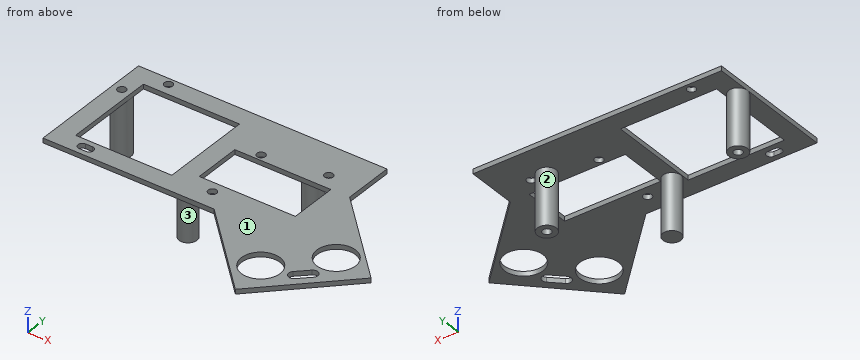
from build123d import *

# Parameters (mm, degrees)
SKETCH_R        = 1.8
SKETCH_W        = 41.028241
SKETCH_H        = 39
SKETCH_W_2      = 41
SKETCH_H_2      = 20.463
PAD_DEPTH       = 2
SKETCH001_R     = 3.8
SKETCH001_R_2   = 4
SKETCH001_R_3   = 1.8
PAD001_DEPTH    = 24
SKETCH002_R     = 8.25
POCKET_DEPTH    = 5
SKETCH003_R     = 1.8
POCKET001_DEPTH = 5


with BuildPart() as part:
    # Sketch → Pad (new body)
    with BuildSketch(Plane.XY):
        Polygon((-53, 15), (53, 15), (53, -6.5), (88.355343, -41.855343), (55.105343, -75.105343), (20, -40), (-53, -40), align=None)
        with Locations((-49, 0)):
            Circle(SKETCH_R, mode=Mode.SUBTRACT)
        with Locations((39.3, 0)):
            Circle(SKETCH_R, mode=Mode.SUBTRACT)
        with Locations((13.2, -31.8)):
            Circle(SKETCH_R, mode=Mode.SUBTRACT)
        with Locations((13.2, -3.8)):
            Circle(SKETCH_R, mode=Mode.SUBTRACT)
        with Locations((-24.485879, -12.5)):
            Rectangle(SKETCH_W, SKETCH_H, mode=Mode.SUBTRACT)
        with Locations((24.528241, -16.768476)):
            Rectangle(SKETCH_W_2, SKETCH_H_2, mode=Mode.SUBTRACT)
        with BuildLine():
            ThreePointArc((-39.199998, -34.2), (-41, -36), (-39.199998, -37.8))
            Line((-39.199998, -37.8), (-36.200009, -37.8))
            ThreePointArc((-36.200009, -37.8), (-34.4, -36.000004), (-36.2, -34.2))
            Line((-39.199998, -34.2), (-36.2, -34.2))
        make_face(mode=Mode.SUBTRACT)
    extrude(amount=PAD_DEPTH)

    # Sketch001 → Pad001 (new body)
    with BuildSketch(Plane(origin=(0, 0, 0), x_dir=(1, 0, 0), z_dir=(0, 0, -1))):
        with Locations((0, 28)):
            Circle(SKETCH001_R)
        with Locations((-49, 0)):
            Circle(SKETCH001_R_2)
        with Locations((-49, 0)):
            Circle(SKETCH001_R_3, mode=Mode.SUBTRACT)
        with Locations((32.6, 0)):
            Circle(SKETCH001_R_2)
        with Locations((32.6, 0)):
            Circle(SKETCH001_R_3, mode=Mode.SUBTRACT)
    extrude(amount=PAD001_DEPTH)

    # Sketch002 → Pocket (cut)
    with BuildSketch(Plane.XY.offset(2)):
        with Locations((53.4328, -58.256155)):
            Circle(SKETCH002_R)
        with Locations((71.433789, -39.081839)):
            Circle(SKETCH002_R)
        with BuildLine():
            ThreePointArc((64.504552, -54.573607), (64.450253, -57.684403), (67.561049, -57.738702))
            Line((67.561049, -57.738702), (72.236758, -53.223423))
            ThreePointArc((72.236758, -53.223423), (72.291056, -50.112627), (69.18026, -50.058329))
            Line((64.504552, -54.573607), (69.18026, -50.058329))
        make_face()
    extrude(amount=-POCKET_DEPTH, mode=Mode.SUBTRACT)

    # Sketch003 → Pocket001 (cut)
    with BuildSketch(Plane.XY.offset(2)):
        with Locations((-38, 12)):
            Circle(SKETCH003_R)
    extrude(amount=-POCKET001_DEPTH, mode=Mode.SUBTRACT)


solid = part.part
Could you check a few things on this model? Use its own coordinates, in mm. Face numbers are marked on the shaded views. Coordinates: 2 decimals unless noted, no trailing zeros. Loops run counter-clockwise (first coordinate to the right, second up) from the corner with the lowest first, then second, coordinate; pieces in that order, holes last.
1. I need wall thicknesses on L1, parallel to Y at x = 13.2, z = 0.5; L2, parallel to Y at x = -38, z = 1.05; L3, parallel to X at y = -1, z = -19. Which ranges of each line are inside material? Lowest first, please.
2. Imagine slicing it at D-D (x = 39.3). Please give me the cut outline in (y, z).
3. For P1, Ø1.6, axis at x = -6, z = 0.5, coming from the -Y side; P2, Ø0.6, axis at y = -16, z = 0.5, coming from the +X side; P3, Ø5, axis at y = -29, z = -14.5, coming from the +X side, each with a flat end and sliding along its axis, tell me the tip position at first contact or that it passes through.
4. Imagine slicing it at C-C (y = -13). Please give me the cut outline in (x, z), and give its area (3 significant figures).
5. Imagine slicing it at B-B (z = -11.75). Please give me the cut outline in (x, y), and give its area (3 significant figures).
6. We'd pull the mould along X, two halves only. Please class the marked faces 1, 2 and 3: released by +X, released by -X, zero draft, split by the parting line, or undercut.
7. Imagine slicing it at A-A (y = 12). Please give me the cut outline in (x, z).
Computed values:
1. L1: y = -40 to -33.6, -30 to -27, -6.54 to -5.6, -2 to 15
1. L2: y = -40 to -37.8, -34.2 to -32, 7 to 10.2, 13.8 to 15
1. L3: x = -52.87 to -50.5, -47.5 to -45.13, 28.73 to 31.1, 34.1 to 36.47
2. outline: (-59.3, 0) - (-27, 0) - (-27, 2) - (-59.3, 2) - close; (-6.54, 0) - (-1.8, 0) - (-1.8, 2) - (-6.54, 2) - close; (1.8, 0) - (15, 0) - (15, 2) - (1.8, 2) - close
3. P1: stops at y = -40
3. P2: stops at x = 62.8
3. P3: stops at x = 3.8
4. outline: (-53, 0) - (-45, 0) - (-45, 2) - (-53, 2) - close; (-3.97, 0) - (4.03, 0) - (4.03, 2) - (-3.97, 2) - close; (45.03, 0) - (59.5, 0) - (59.5, 2) - (45.03, 2) - close
4. area: 60.9 mm2
5. outline: circle Ø8 at (-49, 0); circle Ø7.6 at (0, -28); circle Ø8 at (32.6, 0); hole circle Ø3.6 at (-49, 0); hole circle Ø3.6 at (32.6, 0)
5. area: 126 mm2
6. face 1: zero draft
6. face 2: undercut
6. face 3: split by the parting line
7. outline: (-53, 0) - (-39.8, 0) - (-39.8, 2) - (-53, 2) - close; (-36.2, 0) - (53, 0) - (53, 2) - (-36.2, 2) - close
